```python
from build123d import *

# Parameters (mm, degrees)
EXTRUDE_1_DEPTH           = 70
CUT_EXTRUDE_1_DEPTH       = 100.498743711
SKETCH_3_W                = 10
SKETCH_3_H                = 45
CUT_EXTRUDE_2_DEPTH       = 92.782351245
CUT_EXTRUDE_5_DEPTH       = 92.782351245
CUT_EXTRUDE_6_DEPTH       = 87.740993769
SKETCH_8_W                = 30
SKETCH_8_H                = 32
CUT_EXTRUDE_7_DEPTH       = 27
CUT_EXTRUDE_8_DEPTH       = 84.654049513
SKETCH_10_R               = 2
CUT_EXTRUDE_9_DEPTH       = 27
SKETCH_15_R               = 2.5
CUT_EXTRUDE_11_DEPTH      = 86.399063227
CUT_EXTRUDE_12_DEPTH      = 26
CUT_EXTRUDE_12_DEPTH_BACK = 6
SKETCH_16_R               = 6.5
CHAMFER_1_SIZE            = 1


with BuildPart() as part:
    # 草图1 → 拉伸1 (new body)
    with BuildSketch(Plane.XY):
        Polygon((0, 0), (50, 0), (0, 50), align=None)
    extrude(amount=EXTRUDE_1_DEPTH)

    # 草图2 → 切除-拉伸1 (cut, through all)
    with BuildSketch(Plane.XY.offset(70)):
        Polygon((50, 0), (32, 0), (32, 18), align=None)
    extrude(amount=-CUT_EXTRUDE_1_DEPTH, mode=Mode.SUBTRACT)

    # 草图3 → 切除-拉伸2 (cut, through all)
    with BuildSketch(Plane(origin=(32, 0, 0), x_dir=(0, 0, -1), z_dir=(1, 0, 0))):
        with Locations((-65, 27.5)):
            Rectangle(SKETCH_3_W, SKETCH_3_H)
        with Locations((-45, 27.5)):
            Rectangle(SKETCH_3_W, SKETCH_3_H)
    extrude(amount=-CUT_EXTRUDE_2_DEPTH, mode=Mode.SUBTRACT)

    # 草图6 → 切除-拉伸5 (cut, through all)
    with BuildSketch(Plane.XY.offset(70)):
        Polygon((0, 50), (0, 40), (32, 8), (32, 18), align=None)
    extrude(amount=-CUT_EXTRUDE_5_DEPTH, mode=Mode.SUBTRACT)

    # 草图7 → 切除-拉伸6 (cut, through all)
    with BuildSketch(Plane.XY.offset(70)):
        Polygon((0, 40), (0, 37), (3, 37), align=None)
    extrude(amount=-CUT_EXTRUDE_6_DEPTH, mode=Mode.SUBTRACT)

    # 草图8 → 切除-拉伸7 (cut)
    with BuildSketch(Plane(origin=(32, 0, 0), x_dir=(0, 0, -1), z_dir=(1, 0, 0))):
        with Locations((-15, 21)):
            Rectangle(SKETCH_8_W, SKETCH_8_H)
    extrude(amount=-CUT_EXTRUDE_7_DEPTH, mode=Mode.SUBTRACT)

    # 草图9 → 切除-拉伸8 (cut, through all)
    with BuildSketch(Plane(origin=(5, 0, 0), x_dir=(0, 0, -1), z_dir=(1, 0, 0))):
        Polygon((0, 5), (0, 37), (-30, 37), align=None)
    extrude(amount=-CUT_EXTRUDE_8_DEPTH, mode=Mode.SUBTRACT)

    # 草图10 → 切除-拉伸9 (cut)
    with BuildSketch(Plane.XZ):
        with Locations(Location((6, 65, 0), (0, 0, 270))):
            Circle(SKETCH_10_R)
        with Locations(Location((26, 10, 0), (0, 0, 270))):
            Circle(SKETCH_10_R)
    extrude(amount=-CUT_EXTRUDE_9_DEPTH, mode=Mode.SUBTRACT)

    # 草图15 → 切除-拉伸11 (cut, through all)
    with BuildSketch(Plane.XY.offset(70)):
        with Locations((8, 23)):
            Circle(SKETCH_15_R)
    extrude(amount=-CUT_EXTRUDE_11_DEPTH, mode=Mode.SUBTRACT)

    # 草图16 → 切除-拉伸12 (cut, two sides: drawn at the far end of the back side and taken through both)
    with BuildSketch(Plane(origin=(0, 0, 30), x_dir=(-1, 0, 0), z_dir=(0, 0, -1)).offset(-CUT_EXTRUDE_12_DEPTH_BACK)):
        with Locations((-8, 23)):
            Circle(SKETCH_16_R)
    extrude(amount=CUT_EXTRUDE_12_DEPTH + CUT_EXTRUDE_12_DEPTH_BACK, mode=Mode.SUBTRACT)

    # 倒角1
    chamfer_1_edges = [part.edges().sort_by_distance(p)[0] for p in [
        (0, 37, 35),
        (1.5, 37, 60),
        (1.5, 37, 50),
        (1.5, 37, 40),
        (0, 37, 55),
    ]]
    chamfer(chamfer_1_edges, length=CHAMFER_1_SIZE)


solid = part.part
```
Work out the finished part from the listing and answer in its coordinate system (mm). A direction names the side the tool comes from. Give positions to 0.01 mm unless a question says otherwise; leave off trailing zeros. Write each loop counter-clockwise with the first axis right and the second up, starting at its lowest first coordinate (ties: lowest second). Pieces come first, ordered by that corner, then holes. Notation, with made-up numbers: (-40, 33.5) - (11, 33.5) arc R13 ccw to (11, 51.5) - close; hole circle Ø5 at (-8.75, 62). An arc over 180 degrees is marked (long way). Use one line per item in the form item = value.
1. Each of these flat-tipped pins is pushed along its axis until it touches: pin 1 Ø7 at (y, z) = (32.5, 25) entering from +X; pin 2 Ø6 at (x, y) = (8, 23) entering from +Z; pin 3 Ø3 at (x, z) = (10, 42.5) entering from +Y. Where does it stop, or does it pass through?
Filled in:
pin_1 = 5
pin_2 = 60
pin_3 = 5
2. Consider L1, parallel to X at y = 1, z = 65; L2, parallel to Z at x = 9, y = 12; L3, parallel to Y at x = 13.5, z = 65. Determine where each line is inside the solid, lowest interval first.
Filled in:
L1 = 0 to 4, 8 to 32
L2 = 30 to 40, 50 to 60
L3 = 0 to 5
3. A cutting plane is placed at D-D (x = 9). Write down the section's boundary in (y, z).
Filled in:
outline = (0, 0) - (5, 0) - (5, 30) - (16.58, 30) - (16.58, 36) - (20.71, 36) - (20.71, 40) - (5, 40) - (5, 50) - (20.71, 50) - (20.71, 60) - (5, 60) - (5, 70) - (0, 70) - close; (25.29, 36) - (29.42, 36) - (29.42, 30) - (31, 30) - (31, 40) - (25.29, 40) - close; (25.29, 50) - (31, 50) - (31, 60) - (25.29, 60) - close
4. For faces 1 (the face through (16, 5, 65)), 2 (the face through (16, 11, 30)), 3 (the face through (1.598, 21.875, 29.358)), determine the directions among +Z, -Z, +X, -X, +Y, -Y from which every point of the face is accessible in a straight line to the end or side of a thin tool.
Filled in:
face_1 = +Z, +X, -X, +Y
face_2 = -Z, +X, +Y
face_3 = -Z
5. A cutting plane is placed at A-A (y = 13). Write down the section's boundary in (x, z).
Filled in:
outline = (0, 7.5) - (5, 7.5) - (5, 30) - (27, 30) - (27, 40) - (0, 40) - close; (0, 50) - (27, 50) - (27, 60) - (0, 60) - close
6. A cutting plane is placed at B-B (x = 26). Write down the section's boundary in (y, z), and give its area (3 significant figures).
Filled in:
outline = (0, 0) - (5, 0) - (5, 8) - (0, 8) - close; (0, 12) - (5, 12) - (5, 30) - (14, 30) - (14, 40) - (5, 40) - (5, 50) - (14, 50) - (14, 60) - (5, 60) - (5, 70) - (0, 70) - close
area = 510 mm^2
7. A cutting plane is placed at C-C (z = 65). Write down the section's boundary in (x, y).
Filled in:
outline = (0, 0) - (4, 0) - (4, 5) - (0, 5) - close; (8, 0) - (32, 0) - (32, 5) - (8, 5) - close
8. Determine the mould class of faces 4 (the face through (0, 14, 35)), 5 (the face through (2, 37, 55)), 6 (the face through (9.34, 25.11, 38.03)), 7 (the face through (9.34, 25.11, 55.07)) for opening direction Y: released by +Y, released by -Y, zero draft, split by the parting line, or undercut.
Filled in:
face_4 = zero draft
face_5 = released by +Y
face_6 = undercut
face_7 = undercut
